Autodesk Inventor part; units mm, degrees
ref_plane "YZ Plane" through (0, 0, 0) normal (1, 0, 0) x (0, 1, 0)
ref_plane "XZ Plane" through (0, 0, 0) normal (0, 1, 0) x (-1, 0, 0)
ref_plane "XY Plane" through (0, 0, 0) normal (0, 0, 1) x (1, 0, 0)
sketch "スケッチ1" plane through (0, 0, 0) normal (0, 0, 1) x (1, 0, 0)
  circle A0 centre (0, 0) radius 4
  circle A1 centre (0, 0) radius 2
  dimension "d0" = 8
  dimension "d1" = 4
extrude "押し出し1" add sketch "スケッチ1" against normal blind 1.5 contours A0 | A1
extrude "押し出し2" add sketch "スケッチ1" along normal blind 8 contours A1
sketch "スケッチ2" plane through (0, 0, -1.5) normal (0, 0, -1) x (-1, 0, 0)
  line L0 (-0.5774, 1) -> (0.5774, 1)
  line L1 (0.5774, 1) -> (1.1547, 0)
  line L2 (1.1547, 0) -> (0.5774, -1)
  line L3 (0.5774, -1) -> (-0.5774, -1)
  line L4 (-0.5774, -1) -> (-1.1547, 0)
  line L5 (-1.1547, 0) -> (-0.5774, 1)
  point P0 (0, 0)
  point P1 (0, 0)
  dimension "d6" = 2
extrude "押し出し3" cut sketch "スケッチ2" against normal blind 1.5
chamfer "面取り1" distance 0.5 angle 45 1 edges at (-4, 0, -1.5)
thread "ねじ1"
properties part number "低頭ねじM4×8" material "鋼"
Geometry: final body of the model. Coordinates: model frame, mm. A direction names the side the tool comes from. Round coordinates to 2 decimals unless told otherwise and drop trailing zeros. Order: outer loops, then holes, each group sorted by start corner. A loop starts at its lowest first (then second) coordinate and runs counter-clockwise, first axis right, second up.
Q1. Pin query (flat end, axial travel): pin 1 (1.5 mm diameter, centred on x = 1.5, z = 6, fed in from +Y); pin 2 (1 mm diameter, centred on y = 0, z = 4.5, fed in from -X); pin 3 (1.5 mm diameter, centred on y = -0.5, z = 1.5, fed in from +X). Return the tip coordinate at first contact, or that it passes through.
Result sheet:
pin 1: stops at y = 1.85
pin 2: stops at x = -2
pin 3: stops at x = 2
Q2. Material intervals for probe 1 along Y at (x, z) = (0, 0.25); probe 2 along Y at (x, z) = (0.75, -0.25); probe 3 along Z at (x, y) = (3, 1.25), sorted ascending.
Result sheet:
probe 1: y = -2 to 2
probe 2: y = -3.93 to -0.7, 0.7 to 3.93
probe 3: z = -1.5 to 0
Q3. Access query for faces 4 (the face through (0, 2, 4)), 5 (the face through (0, 0, 0)), 6 (the face through (0, 0, 8)). Directions: +Z, -Z, +X, -X, +Y, -Y. A direction counts if a zero-diameter tool reaches every point of the face in a straight line with its end or side. Return the directions, or none.
Result sheet:
face 4: +Z
face 5: -Z
face 6: +Z, +X, -X, +Y, -Y
Q4. Section A-A, the plane x = 0. Output: boundary loops of the cut face in (y, z).
Result sheet:
outline: (-4, -1) - (-3.5, -1.5) - (-1, -1.5) - (-1, 0) - (1, 0) - (1, -1.5) - (3.5, -1.5) - (4, -1) - (4, 0) - (2, 0) - (2, 8) - (-2, 8) - (-2, 0) - (-4, 0) - close
Q5. Mould query, pull axis X, two halves, no side actions, for faces 1 (the face through (-0.867, -3.905, -0.493)), 2 (the face through (-0.86, 0.51, -0.76)), 3 (the face through (1, 1, -1.5)). Classes: released by +X, released by -X, zero draft, split by the parting line, or undercut.
Result sheet:
face 1: split by the parting line
face 2: undercut
face 3: zero draft
Q6. Section B-B, the plane z = 2. Output: boundary loops of the cut face in (x, y).
Result sheet:
outline: circle Ø4 at (0, 0)
